Design review of the part built by this model. Coordinates are the model's own, in mm. Face numbers are marked on the shaded views. A direction names the side the tool comes from. Give positions to 0.01 mm unless a question says otherwise; leave off trailing zeros. Order: outer loops, then holes, each group sorted by start corner. A loop starts at its lowest first (then second) coordinate and runs counter-clockwise, first axis right, second up. Notation, with made-up numbers: M 77.5,-34 L 122.5,-34 A19 cw 122.5,-20 Z; hole C 1.25,34 d2. An arc over 180 degrees is marked long. Put each result on its own line as item: value. Start each with the question number.
from build123d import *

# Parameters (mm, degrees)
BRIDA_BASE1_DEPTH                  = 19.5
BRIDA_DE_ARISTA1_STRIP_W           = 3
BRIDA_DE_ARISTA1_STRIP_H           = 0.5
BRIDA_DE_ARISTA1_STRIP_CUT_DEPTH   = 15.5
BRIDA_DE_ARISTA1_STRIP_2_W         = 3
BRIDA_DE_ARISTA1_STRIP_2_H         = 0.5
BRIDA_DE_ARISTA1_STRIP_CUT_2_DEPTH = 15.5
BRIDA_DE_ARISTA1_DEPTH             = 15.5
BRIDA_DE_ARISTA1_BEND_DEPTH        = 15.5
CROQUIS11_R                        = 3
CORTAR_EXTRUIR1_DEPTH              = 57.369658542
CROQUIS14_R                        = 1
CORTAR_EXTRUIR2_DEPTH              = 10
CROQUIS15_R                        = 1.5
CORTAR_EXTRUIR3_DEPTH              = 10
CROQUIS16_R                        = 1.5
CORTAR_EXTRUIR4_DEPTH              = 0.5


# Sheet-metal steps are written as plain solids
with BuildPart() as part:
    # Croquis1 → Brida base1 (new body)
    with BuildSketch(Plane(origin=(0, 0, 0), x_dir=(0, 0, -1), z_dir=(1, 0, 0))):
        with BuildLine():
            Line((-35.363451777, 5.587428088), (-35.363451777, -9.912571912))
            ThreePointArc((-35.363451777, -9.912571912), (-35.217005167, -10.266125303), (-34.863451777, -10.412571912))
            Line((-34.863451777, -10.412571912), (26.136548223, -10.412571912))
            ThreePointArc((26.136548223, -10.412571912), (26.490101614, -10.266125303), (26.636548223, -9.912571912))
            Line((26.636548223, -9.912571912), (26.636548223, 5.587428088))
            Line((26.636548223, 5.587428088), (27.136548223, 5.587428088))
            Line((27.136548223, 5.587428088), (27.136548223, -9.912571912))
            ThreePointArc((27.136548223, -9.912571912), (26.843655005, -10.619678693), (26.136548223, -10.912571912))
            Line((26.136548223, -10.912571912), (-34.863451777, -10.912571912))
            ThreePointArc((-34.863451777, -10.912571912), (-35.570558558, -10.619678693), (-35.863451777, -9.912571912))
            Line((-35.863451777, -9.912571912), (-35.863451777, 5.587428088))
            Line((-35.863451777, 5.587428088), (-35.363451777, 5.587428088))
        make_face()
    extrude(amount=BRIDA_BASE1_DEPTH)

    # Brida de arista1 strip (across the edge) → Brida de arista1 strip cut (cut)
    with BuildSketch(Plane(origin=(19.5, -9.912571912, 35.863451777), x_dir=(-1, 0, 0), z_dir=(0, 1, 0))):
        with Locations((-1, -0.25)):
            Rectangle(BRIDA_DE_ARISTA1_STRIP_W, BRIDA_DE_ARISTA1_STRIP_H)
    extrude(amount=BRIDA_DE_ARISTA1_STRIP_CUT_DEPTH, mode=Mode.SUBTRACT)

    # Brida de arista1 strip 2 (across the edge) → Brida de arista1 strip cut 2 (cut)
    with BuildSketch(Plane(origin=(0, 5.587428088, 35.863451777), x_dir=(1, 0, 0), z_dir=(0, -1, 0))):
        with Locations((-1, -0.25)):
            Rectangle(BRIDA_DE_ARISTA1_STRIP_2_W, BRIDA_DE_ARISTA1_STRIP_2_H)
    extrude(amount=BRIDA_DE_ARISTA1_STRIP_CUT_2_DEPTH, mode=Mode.SUBTRACT)

    # Brida de arista1 section (across the edge) → Brida de arista1 (add)
    with BuildSketch(Plane(origin=(19.5, -9.912571912, 35.863451777), x_dir=(-1, 0, 0), z_dir=(0, 1, 0))):
        with BuildLine():
            Line((-0.5, 0.5), (-0.5, 15.5))
            Line((-0.5, 15.5), (0, 15.5))
            Line((0, 15.5), (0, 0.5))
            ThreePointArc((0, 0.5), (0.146446609, 0.146446609), (0.5, 0))
            Line((0.5, 0), (0.5, -0.5))
            ThreePointArc((0.5, -0.5), (-0.207106781, -0.207106781), (-0.5, 0.5))
        make_face()
    extrude(amount=BRIDA_DE_ARISTA1_DEPTH)

    # Brida de arista1 section 2 (across the edge) → Brida de arista1 bend (add)
    with BuildSketch(Plane(origin=(0, 5.587428088, 35.863451777), x_dir=(1, 0, 0), z_dir=(0, -1, 0))):
        with BuildLine():
            Line((-0.5, 0.5), (-0.5, 15.5))
            Line((-0.5, 15.5), (0, 15.5))
            Line((0, 15.5), (0, 0.5))
            ThreePointArc((0, 0.5), (0.146446609, 0.146446609), (0.5, 0))
            Line((0.5, 0), (0.5, -0.5))
            ThreePointArc((0.5, -0.5), (-0.207106781, -0.207106781), (-0.5, 0.5))
        make_face()
    extrude(amount=BRIDA_DE_ARISTA1_BEND_DEPTH)

    # Croquis11 → Cortar-Extruir1 (cut, through all)
    with BuildSketch(Plane(origin=(20, 0, 0), x_dir=(0, 0, -1), z_dir=(1, 0, 0))):
        with Locations(Location((-43.613451777, -2.162571912, 0), (0, 0, 180))):
            Circle(CROQUIS11_R)
        with BuildLine():
            ThreePointArc((-43.613451777, -9.912571912), (-49.093529331, -7.642649466), (-51.363451777, -2.162571912))
            Line((-51.363451777, -2.162571912), (-51.363451777, -9.912571912))
            Line((-51.363451777, -9.912571912), (-43.613451777, -9.912571912))
        make_face()
        with BuildLine():
            ThreePointArc((-51.363451777, -2.162571912), (-49.093529331, 3.317505642), (-43.613451777, 5.587428088))
            Line((-43.613451777, 5.587428088), (-51.363451777, 5.587428088))
            Line((-51.363451777, 5.587428088), (-51.363451777, -2.162571912))
        make_face()
    extrude(amount=-CORTAR_EXTRUIR1_DEPTH, mode=Mode.SUBTRACT)

    # Croquis14 → Cortar-Extruir2 (cut)
    with BuildSketch(Plane.XY.offset(35.863451777)):
        with Locations((15.21, -2.162571912)):
            Circle(CROQUIS14_R)
        with Locations((4.29, -2.162571912)):
            Circle(CROQUIS14_R)
        with BuildLine():
            Line((6.25, 5.587428088), (6.25, -2.162571912))
            ThreePointArc((6.25, -2.162571912), (9.75, -5.662571912), (13.25, -2.162571912))
            Line((13.25, -2.162571912), (13.25, 5.587428088))
            Line((13.25, 5.587428088), (6.25, 5.587428088))
        make_face()
    extrude(amount=-CORTAR_EXTRUIR2_DEPTH, mode=Mode.SUBTRACT)

    # Croquis15 → Cortar-Extruir3 (cut)
    with BuildSketch(Plane(origin=(0, 0, -27.136548223), x_dir=(-1, 0, 0), z_dir=(0, 0, -1))):
        with Locations((-13.75, -2.162571912)):
            Circle(CROQUIS15_R)
        with Locations(Location((-5.75, -2.162571912, 0), (0, 0, 180))):
            Circle(CROQUIS15_R)
    extrude(amount=-CORTAR_EXTRUIR3_DEPTH, mode=Mode.SUBTRACT)

    # Croquis16 → Cortar-Extruir4 (cut)
    with BuildSketch(Plane(origin=(0, -10.412571912, 0), x_dir=(-1, 0, 0), z_dir=(0, 1, 0))):
        with Locations(Location((-9.75, -18.636548223, 0), (0, 0, 90))):
            Circle(CROQUIS16_R)
        with BuildLine():
            Line((-3.747619635, -21.636548223), (-15.752380365, -21.636548223))
            ThreePointArc((-15.752380365, -21.636548223), (-17.252380365, -23.136548223), (-15.752380365, -24.636548223))
            Line((-15.752380365, -24.636548223), (-3.747619635, -24.636548223))
            ThreePointArc((-3.747619635, -24.636548223), (-2.247619635, -23.136548223), (-3.747619635, -21.636548223))
        make_face()
    extrude(amount=-CORTAR_EXTRUIR4_DEPTH, mode=Mode.SUBTRACT)


solid = part.part
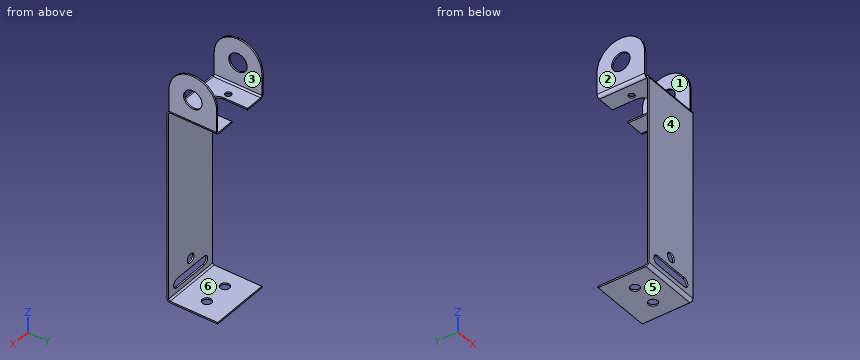
1. Consider section B-B on y = 2. Give the boundary of the cut face in (x, z), then the cut area to 3 significant figures.
2. To check wall thickness, follow probe 1 along Z at (x, y) = (14.75, 3); probe 2 along X at (y, z) = (-5, 36.5); probe 3 along Y at (x, z) = (16.75, -1). State the ranges of each line that lie inside material, in increasing order.
3. The part is to be moulded in two halves that separate along X. For the marked faces 1, 2, 3 and 4, say which applies: +X half, -X half, draft (parallel to the pull), parting line (faces both ways), or undercut.
4. Consider section A-A on x = 9.75. Give the boundary of the cut face in (y, z).
5. Machinability: for the marked faces 5 and 6, which of the approach directions +Z, -Z, +X, -X, +Y, -Y give a long, thin tool a straight path to every point of the face, cutting with its end or side? Answer none if there is none.
6. Insertion check: pin 1 (1.5 mm diameter, centred on x = 15.5, y = -3.5, fed in from +Z); pin 2 (10 mm diameter, centred on x = 11.5, z = 9.5, fed in from +Y); pin 3 (1.8 mm diameter, centred on x = 4.29, y = -2.16, fed in from +Z). Each pin has a flat end and moves straight along its axis. Give the tip position at first contact, or say it passes through.
7. Consider section C-C on x = 1.25. Give the boundary of the cut face in (y, z), then the cut area to 3 significant figures.
8. Consider section D-D on z = 20. Give the boundary of the cut face in (x, y), then the cut area to 3 significant figures.
Returned:
1. outline: M -0.5,36.36 A1 ccw 0.5,35.36 L 6.25,35.36 L 6.25,35.86 L 0.5,35.86 A0.5 cw 0,36.36 L 0,50.15 L -0.5,50.15 Z; M 0,-27.14 L 19.5,-27.14 L 19.5,-26.64 L 0,-26.64 Z; M 13.25,35.36 L 19,35.36 A1 ccw 20,36.36 L 20,50.15 L 19.5,50.15 L 19.5,36.36 A0.5 cw 19,35.86 L 13.25,35.86 Z
1. area: 30.5 mm2
2. probe 1: z = -27.14 to -26.64, 35.36 to 35.86
2. probe 2: x = -0.5 to 0, 19.5 to 20
2. probe 3: y = -10.91 to -10.41
3. face 1: undercut
3. face 2: -X half
3. face 3: undercut
3. face 4: draft
4. outline: M -10.91,-26.14 A1 ccw -9.91,-27.14 L 5.59,-27.14 L 5.59,-26.64 L -9.91,-26.64 A0.5 cw -10.41,-26.14 L -10.41,-24.64 L -10.91,-24.64 Z; M -10.91,-21.64 L -10.41,-21.64 L -10.41,-20.14 L -10.91,-20.14 Z; M -10.91,-17.14 L -10.41,-17.14 L -10.41,34.86 A0.5 cw -9.91,35.36 L -5.66,35.36 L -5.66,35.86 L -9.91,35.86 A1 ccw -10.91,34.86 Z
5. face 5: -Z, +X, -X, +Y, -Y
5. face 6: +X, -X, +Y
6. pin 1: stops at z = 35.86
6. pin 2: stops at y = -10.41
6. pin 3: stops at z = -26.64
7. outline: M -10.91,-26.14 A1 ccw -9.91,-27.14 L 5.59,-27.14 L 5.59,-26.64 L -9.91,-26.64 A0.5 cw -10.41,-26.14 L -10.41,34.86 A0.5 cw -9.91,35.36 L 5.59,35.36 L 5.59,35.86 L -9.91,35.86 A1 ccw -10.91,34.86 Z
7. area: 47.2 mm2
8. outline: M 0,-10.91 L 19.5,-10.91 L 19.5,-10.41 L 0,-10.41 Z
8. area: 9.75 mm2
